Check sheet for the modelled part. Datum: model origin and axes. Units: mm. Face numbers are marked on the shaded views. A direction names the side the tool comes from. Coordinates: 2 decimals unless noted, no trailing zeros. Loops run counter-clockwise (first coordinate to the right, second up) from the corner with the lowest first, then second, coordinate; pieces in that order, holes last. Notation, with made-up numbers: M 51,-10 L 101,-10 A11 ccw 101,4 Z; hole C 76,87 d7. An arc over 180 degrees is marked long. Answer in a Markdown table with one row per item. Add a question column.
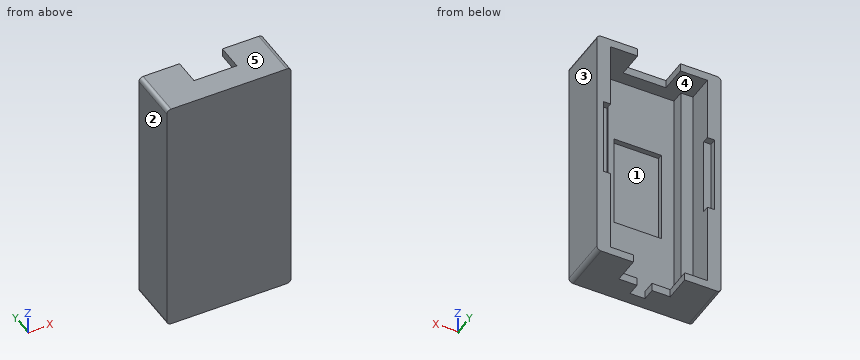
```python
from build123d import *

# Parameters (mm, degrees)
SKETCH2_W           = 29
SKETCH2_H           = 57
BOSS_EXTRUDE1_DEPTH = 12
SKETCH3_W           = 22.6
SKETCH3_H           = 53.2
CUT_EXTRUDE1_DEPTH  = 6.2
SKETCH4_W           = 17
SKETCH4_H           = 53.2
CUT_EXTRUDE2_DEPTH  = 3
SKETCH5_W           = 11.1
SKETCH5_H           = 22.1
CUT_EXTRUDE3_DEPTH  = 1.2
SKETCH6_W           = 26
SKETCH6_H           = 18.5
CUT_EXTRUDE4_DEPTH  = 1.6
SKETCH7_W           = 12
SKETCH7_H           = 1.9
SKETCH7_W_2         = 10
CUT_EXTRUDE5_DEPTH  = 6.2
FILLET1_R           = 1
SKETCH8_W           = 3.5
SKETCH8_H           = 3
CUT_EXTRUDE6_DEPTH  = 10


with BuildPart() as part:
    # Sketch2 → Boss-Extrude1 (new body)
    with BuildSketch(Plane(origin=(0, 0, 0), x_dir=(1, 0, 0), z_dir=(0, 1, 0))):
        Rectangle(SKETCH2_W, SKETCH2_H)
    extrude(amount=BOSS_EXTRUDE1_DEPTH)

    # Sketch3 → Cut-Extrude1 (cut)
    with BuildSketch(Plane(origin=(0, 12, 0), x_dir=(1, 0, 0), z_dir=(0, 1, 0))):
        Rectangle(SKETCH3_W, SKETCH3_H)
    extrude(amount=-CUT_EXTRUDE1_DEPTH, mode=Mode.SUBTRACT)

    # Sketch4 → Cut-Extrude2 (cut)
    with BuildSketch(Plane(origin=(0, 5.8, 0), x_dir=(1, 0, 0), z_dir=(0, 1, 0))):
        Rectangle(SKETCH4_W, SKETCH4_H)
    extrude(amount=-CUT_EXTRUDE2_DEPTH, mode=Mode.SUBTRACT)

    # Sketch5 → Cut-Extrude3 (cut)
    with BuildSketch(Plane(origin=(0, 2.8, 0), x_dir=(1, 0, 0), z_dir=(0, 1, 0))):
        Rectangle(SKETCH5_W, SKETCH5_H)
    extrude(amount=-CUT_EXTRUDE3_DEPTH, mode=Mode.SUBTRACT)

    # Sketch6 → Cut-Extrude4 (cut)
    with BuildSketch(Plane(origin=(0, 12, 0), x_dir=(1, 0, 0), z_dir=(0, 1, 0))):
        with Locations((0, -2.15)):
            Rectangle(SKETCH6_W, SKETCH6_H)
    extrude(amount=-CUT_EXTRUDE4_DEPTH, mode=Mode.SUBTRACT)

    # Sketch7 → Cut-Extrude5 (cut)
    with BuildSketch(Plane(origin=(0, 12, 0), x_dir=(1, 0, 0), z_dir=(0, 1, 0))):
        with Locations((0, 27.55)):
            Rectangle(SKETCH7_W, SKETCH7_H)
        with Locations((0, -27.55)):
            Rectangle(SKETCH7_W_2, SKETCH7_H)
    extrude(amount=-CUT_EXTRUDE5_DEPTH, mode=Mode.SUBTRACT)

    # Fillet1
    fillet1_edges = [part.edges().sort_by_distance(p)[0] for p in [
        (14.5, 6, 28.5),
        (-14.5, 6, 28.5),
        (-14.5, 6, -28.5),
        (14.5, 6, -28.5),
    ]]
    fillet(fillet1_edges, radius=FILLET1_R)

    # Sketch8 → Cut-Extrude6 (cut)
    with BuildSketch(Plane(origin=(0, 0, -28.5), x_dir=(-1, 0, 0), z_dir=(0, 0, -1))):
        with Locations((0, 4.3)):
            Rectangle(SKETCH8_W, SKETCH8_H)
    extrude(amount=-CUT_EXTRUDE6_DEPTH, mode=Mode.SUBTRACT)


solid = part.part
```
Q1. Cross-section at C-C (z = 21). Record the cut outline in (x, y).
Q2. Cross-section at A-A (x = -4.25). Record the cut outline in (y, z), plus the area to 3 significant figures.
Q3. Cross-section at B-B (y = 9.75). Record the cut outline in (x, z).
Q4. Cross-section at D-D (y = 4.75). Record the cut outline in (x, z), plus the area to 3 significant figures.
Q5. Go/stop test with flat-tipped pins: pin 1 (9 mm diameter, centred on x = 0.5, z = -2, fed in from +Y); pin 2 (0.9 mm diameter, centred on x = -0.5, z = 27.5, fed in from +Y); pin 3 (5 mm diameter, centred on x = -3.5, z = -8.5, fed in from +Y). Record where each tip stops, or that it passes through.
Q6. Access from +Z, -Z, +X, -X, +Y, -Y to the whole of each face (thin tool, end or side, straight path). Record for the marked faces 1 and 2.
Q7. Mould release check, pull along X, two halves, no side actions. Record for the marked faces 3, 4 and 5: released by +X, released by -X, zero draft, split by the parting line, or undercut.
Q8. Thickness scan on L1, parallel to Z at x = 3.75, y = 4.5; L2, parallel to X at y = 7.5, z = 5; L3, parallel to X at y = 4, z = 18. Record the ranges inside material, lowest first.
Answer key:
| question | item | result |
|---|---|---|
| 1 | outline | M -14.5,0 L 14.5,0 L 14.5,12 L 11.3,12 L 11.3,5.8 L 8.5,5.8 L 8.5,2.8 L -8.5,2.8 L -8.5,5.8 L -11.3,5.8 L -11.3,12 L -14.5,12 Z |
| 2 | outline | M 0,-28.5 L 5.8,-28.5 L 5.8,-26.6 L 2.8,-26.6 L 2.8,-11.05 L 1.6,-11.05 L 1.6,11.05 L 2.8,11.05 L 2.8,26.6 L 5.8,26.6 L 5.8,28.5 L 0,28.5 Z |
| 2 | area | 144 mm^2 |
| 3 | outline | M -14.5,-27.5 A1 ccw -13.5,-28.5 L -6,-28.5 L -6,-26.6 L -11.3,-26.6 L -11.3,26.6 L -5,26.6 L -5,28.5 L -13.5,28.5 A1 ccw -14.5,27.5 Z; M 5,26.6 L 11.3,26.6 L 11.3,-26.6 L 6,-26.6 L 6,-28.5 L 13.5,-28.5 A1 ccw 14.5,-27.5 L 14.5,27.5 A1 ccw 13.5,28.5 L 5,28.5 Z |
| 4 | outline | M -14.5,-27.5 A1 ccw -13.5,-28.5 L -1.75,-28.5 L -1.75,-26.6 L -8.5,-26.6 L -8.5,26.6 L 8.5,26.6 L 8.5,-26.6 L 1.75,-26.6 L 1.75,-28.5 L 13.5,-28.5 A1 ccw 14.5,-27.5 L 14.5,27.5 A1 ccw 13.5,28.5 L -13.5,28.5 A1 ccw -14.5,27.5 Z |
| 4 | area | 741 mm^2 |
| 5 | pin 1 | y = 1.6 |
| 5 | pin 2 | y = 5.8 |
| 5 | pin 3 | y = 2.8 |
| 6 | face 1 | +Y |
| 6 | face 2 | +Z, -Z, -X, +Y, -Y |
| 7 | face 3 | released by +X |
| 7 | face 4 | undercut |
| 7 | face 5 | zero draft |
| 8 | L1 | -28.5 to -26.6, 26.6 to 28.5 |
| 8 | L2 | -14.5 to -11.3, 11.3 to 14.5 |
| 8 | L3 | -14.5 to -8.5, 8.5 to 14.5 |
